Autodesk Fusion 360 part; units mm, degrees
sketch "Sketch2" plane through (0, 0, 0) normal (0, 0, 1) x (1, 0, 0)
  circle A0 centre (0, 0) radius 45 construction
  line L0 (-28.5, 3.7528) -> (-35, 7.5056)
  line L1 (-35, 7.5056) -> (-41.5, 3.7528)
  line L2 (-41.5, 3.7528) -> (-41.5, -3.7528)
  line L3 (-41.5, -3.7528) -> (-35, -7.5056)
  line L4 (-35, -7.5056) -> (-28.5, -3.7528)
  line L5 (-28.5, -3.7528) -> (-28.5, 3.7528)
  line L6 (11.0007, -26.557) -> (10.9993, -34.0625)
  line L7 (10.9993, -34.0625) -> (17.4987, -37.8164)
  line L8 (17.4987, -37.8164) -> (23.9993, -34.0648)
  line L9 (23.9993, -34.0648) -> (24.0007, -26.5592)
  line L10 (24.0007, -26.5592) -> (17.5013, -22.8053)
  line L11 (17.5013, -22.8053) -> (11.0007, -26.557)
  line L12 (17.5, 22.8053) -> (24, 26.5581)
  line L13 (24, 26.5581) -> (24, 34.0637)
  line L14 (24, 34.0637) -> (17.5, 37.8164)
  line L15 (17.5, 37.8164) -> (11, 34.0637)
  line L16 (11, 34.0637) -> (11, 26.5581)
  line L17 (11, 26.5581) -> (17.5, 22.8053)
  circle A1 centre (0, 0) radius 4
  circle A2 centre (0, 0) radius 6.075
  circle A3 centre (0, 0) radius 9.6
  line L18 (-8.0769, -13.9896) -> (-36.4286, -9.8974)
  line L19 (-8.0769, 13.9896) -> (-36.4286, 9.8974)
  line L20 (16.1538, 0) -> (26.7857, -26.5994)
  line L21 (-8.0769, -13.9896) -> (9.6429, -36.4968)
  line L22 (-8.0769, 13.9896) -> (9.6429, 36.4968)
  line L23 (16.1538, 0) -> (26.7857, 26.5994)
  arc A4 (-36.4286, 9.8974) -> (-36.4286, -9.8974) centre (-35, 0) ccw
  arc A5 (26.7857, 26.5994) -> (9.6429, 36.4968) centre (17.5, 30.3109) ccw
  arc A6 (9.6429, -36.4968) -> (26.7857, -26.5994) centre (17.5, -30.3109) ccw
  point P0 (-35, 0)
  point P1 (17.5, -30.3109)
  point P2 (17.5, 30.3109)
  dimension "d1" = 90
  dimension "d3" = 6.5
  dimension "d4" = 35
  dimension "d7" = 6.5
  dimension "d8" = 6.5
  dimension "d9" = 8
  dimension "d10" = 12.15
  dimension "d11" = 19.2
  dimension "d12" = 35
  dimension "d13" = 35
extrude "Extrude1" add sketch "Sketch2" along normal mid plane 8 contours L18 L19 L20 L21 L22 L23 A4 A5 A6
fillet "Fillet1" radius 5 3 edges at (-8.0769, -13.9896, 0) (16.1538, 0, 0) (-8.0769, 13.9896, 0)
chamfer "Chamfer1" distance 2 angle 45 12 edges at (-8.2692, 14.3227, 4) (-23.2418, 11.8008, 4) (-45, 0, 4) (-23.2418, -11.8008, 4) (-8.2692, -14.3227, 4) (1.4011, -26.0283, 4) (22.5, -38.9711, 4) (21.8407, -14.2276, 4) (16.5385, 0, 4) (21.8407, 14.2276, 4) (22.5, 38.9711, 4) (1.4011, 26.0283, 4)
chamfer "Chamfer2" distance 2 angle 45 12 edges at (21.8407, 14.2276, -4) (16.5385, 0, -4) (21.8407, -14.2276, -4) (22.5, -38.9711, -4) (1.4011, -26.0283, -4) (-8.2692, -14.3227, -4) (-23.2418, -11.8008, -4) (-45, 0, -4) (-23.2418, 11.8008, -4) (-8.2692, 14.3227, -4) (1.4011, 26.0283, -4) (22.5, 38.9711, -4)
The model under review builds one solid part; all positions refer to its coordinate system, in mm. A direction names the side the tool comes from. Round coordinates to 2 decimals unless told otherwise and drop trailing zeros. Write each loop counter-clockwise with the first axis right and the second up, starting at its lowest first coordinate (ties: lowest second). Pieces come first, ordered by that corner, then holes. Notation, with made-up numbers: (4.25, 4) - (48.25, 4) arc R22 cw to (48.25, 21) - close; hole circle Ø5 at (-0.5, 83.5). An arc over 180 degrees is marked (long way). One line per item, written item: value. Start each with the question number.
1. Machinability: for faces 5 (the face through (-31.7, 5.6, -0.1)), 6 (the face through (-7.7, -13.5, 3)), 7 (the face through (20.856, 14.42, -2.986)), which of the approach directions +Z, -Z, +X, -X, +Y, -Y give a long, thin tool a straight path to every point of the face, cutting with its end or side? Answer none if there is none.
2. Consider section C-C on x = -32. Write out the cut boundary in (y, z), and give its area (3 significant figures).
3. Consider section B-B on z = 0.75. State how many separate pieces and enclosed holes the cut face has, and give its area (3 significant figures).
4. Clearance check with flat-ended pins moving along their axes: P1, Ø15.5, axis at x = 0, y = 0, coming from the -Z side; P2, Ø4, axis at y = -0.5, z = 1, coming from the -X side; P3, Ø4, axis at x = 0, z = 3, coming from the +Y side; P4, Ø4, axis at x = -13.5, z = 2, coming from the +Y side. State where each tip first meets the part, or that it passes through.
5. To check wall thickness, follow L1, parallel to Y at x = 0, z = 1; L2, parallel to X at y = -1, z = 0.5; L3, parallel to X at y = -0.5, z = -2. State the ranges of each line that lie inside material, in increasing order. Write a range as from..to.
6. The part is to be moulded in two halves that separate along Y. For faces 1 (the face through (6, 9, -4)), 2 (the face through (5.161, -8.095, -0.056)), 3 (the face through (1.3, 25.9, 0)), 4 (the face through (-43.123, -0.162, 3.875)), say which applies: released by +Y, released by -Y, zero draft, split by the parting line, or undercut.
7. Consider section A-A on y = 0. Write out the cut boundary in (x, z), and give its area (3 significant figures).
8. Consider section D-D on x = -20. Write out the cut boundary in (y, z).
Checks:
1. face 5: +Z, -Z
1. face 6: +Z, -X, -Y
1. face 7: -Z, +X
2. outline: (-10.54, -2) - (-8.52, -4) - (-5.77, -4) - (-5.77, 4) - (-8.52, 4) - (-10.54, 2) - close; (5.77, -4) - (8.52, -4) - (10.54, -2) - (10.54, 2) - (8.52, 4) - (5.77, 4) - close
2. area: 68.1 mm^2
3. separate pieces: 1
3. enclosed holes: 4
3. area: 2,030 mm^2
4. P1: passes through
4. P2: stops at x = -45
4. P3: stops at y = 26.45
4. P4: stops at y = 13.5
5. L1: y = -24.25..-9.6, 9.6..24.25
5. L2: x = -44.95..-41.5, -28.5..-9.55, 9.55..16.64
5. L3: x = -44.99..-41.5, -28.5..-9.59, 9.59..16.56
6. face 1: zero draft
6. face 2: undercut
6. face 3: released by +Y
6. face 4: split by the parting line
7. outline: (-45, -2) - (-43, -4) - (-41.5, -4) - (-41.5, 4) - (-43, 4) - (-45, 2) - close; (-28.5, -4) - (-9.6, -4) - (-9.6, 4) - (-28.5, 4) - close; (9.6, -4) - (14.54, -4) - (16.54, -2) - (16.54, 2) - (14.54, 4) - (9.6, 4) - close
7. area: 227 mm^2
8. outline: (-12.27, -2) - (-10.25, -4) - (10.25, -4) - (12.27, -2) - (12.27, 2) - (10.25, 4) - (-10.25, 4) - (-12.27, 2) - close
